Autodesk Inventor part; units mm, degrees
ref_plane "YZ Plane" through (0, 0, 0) normal (1, 0, 0) x (0, 1, 0)
ref_plane "XZ Plane" through (0, 0, 0) normal (0, 1, 0) x (-1, 0, 0)
ref_plane "XY Plane" through (0, 0, 0) normal (0, 0, 1) x (1, 0, 0)
sketch "Sketch1" plane through (0, 0, 0) normal (0, 0, 1) x (1, 0, 0)
  line L0 (13.75, -9.25) -> (-13.75, -9.25)
  line L1 (-13.75, -9.25) -> (-13.75, 9.25)
  line L2 (-13.75, 9.25) -> (13.75, 9.25)
  line L3 (13.75, 9.25) -> (13.75, -9.25)
  line L4 (13.75, -9.25) -> (-13.75, 9.25) construction
  line L5 (-13.75, -9.25) -> (13.75, 9.25) construction
  line L6 (-16, 0) -> (16, 0) construction
  circle A0 centre (-16, 0) radius 4
  circle A1 centre (16, 0) radius 4
  line L7 (30, -1) -> (-30, -1)
  line L8 (-30, -1) -> (-30, 1)
  line L9 (-30, 1) -> (30, 1)
  line L10 (30, 1) -> (30, -1)
  line L11 (30, -1) -> (-30, 1) construction
  line L12 (-30, -1) -> (30, 1) construction
  line L13 (30, -6.5) -> (-30, -6.5)
  line L14 (-30, -6.5) -> (-30, 6.5)
  line L15 (-30, 6.5) -> (30, 6.5)
  line L16 (30, 6.5) -> (30, -6.5)
  line L17 (30, -6.5) -> (-30, 6.5) construction
  line L18 (-30, -6.5) -> (30, 6.5) construction
  point P0 (0, 0)
  point P1 (-19.873, -1)
  point P2 (-13.75, -6.5)
  point P3 (13.75, -6.5)
  point P4 (19.873, -1)
  point P5 (19.873, 1)
  point P6 (13.75, 6.5)
  point P7 (-13.75, 6.5)
  point P8 (-19.873, 1)
  dimension "d0" = 27.5
  dimension "d1" = 18.5
  dimension "d2" = 8
  dimension "d3" = 8
  dimension "d4" = 32
  dimension "d5" = 60
  dimension "d6" = 2
  dimension "d7" = 13
extrude "Extrusion1" add sketch "Sketch1" along normal blind 6.35 contours L0 L1 L13 L3 | L13 L1 A0 L7 A1 L3 | L3 A1 L7 L16 L13 | L13 L14 L7 A0 L1 | L7 A0 L9 A1 | L9 A0 L1 L15 L3 A1 | L9 A1 L3 L15 L16 | L9 L14 L15 L1 A0 | L15 L1 L2 L3
fillet "Fillet4" radius 3 4 edges at (-19.873, 1, 3.175) (-19.873, -1, 3.175) (19.873, 1, 3.175) (19.873, -1, 3.175)
fillet "Fillet1" radius 2 4 edges at (13.75, 9.25, 3.175) (-13.75, 9.25, 3.175) (-13.75, -9.25, 3.175) (13.75, -9.25, 3.175)
fillet "Fillet2" radius 2 4 edges at (-30, 6.5, 3.175) (-30, -6.5, 3.175) (30, 6.5, 3.175) (30, -6.5, 3.175)
fillet "Fillet3" radius 1 8 edges at (-30, -1, 3.175) (-30, 1, 3.175) (-13.75, -6.5, 3.175) (-13.75, 6.5, 3.175) (13.75, 6.5, 3.175) (13.75, -6.5, 3.175) (30, 1, 3.175) (30, -1, 3.175)
sketch "Sketch2" plane through (0, 0, 6.35) normal (0, 0, 1) x (1, 0, 0)
  line L0 (10, -5.5) -> (-10, -5.5) construction
  line L1 (-10, -5.5) -> (-10, 5.5) construction
  line L2 (-10, 5.5) -> (10, 5.5) construction
  line L3 (10, 5.5) -> (10, -5.5) construction
  line L4 (10, -5.5) -> (-10, 5.5) construction
  line L5 (-10, -5.5) -> (10, 5.5) construction
  circle A0 centre (-10, 5.5) radius 3 construction
  circle A1 centre (-10, -5.5) radius 3 construction
  circle A2 centre (-10, 5.5) radius 1.65 construction
  line L6 (11.75, 9.25) -> (-11.75, 9.25) construction
  point P0 (0, 0)
  dimension "d13" = 20
  dimension "d14" = 11
  dimension "d22" = 6
  dimension "d23" = 6
  dimension "d25" = 3.3
  dimension "d26" = 2.1
hole "Hole1" at (-10, 5.5, 6.35) at (10, 5.5, 6.35) at (10, -5.5, 6.35) at (-10, -5.5, 6.35) direction (0, 0, -1) diameter 3.3 end through all
sketch "Sketch3" plane through (0, 0, 6.35) normal (0, 0, 1) x (1, 0, 0)
  point P0 (0, 0)
hole "Hole2" at (0, 0, 6.35) direction (0, 0, -1) diameter 3.3 end through all
properties part number "Printhead Belt Retainer R2" material "Aluminum 6061"
Can you work these out from the model? Positions are in its coordinate system, mm. A direction names the side the tool comes from. Coordinates: 2 decimals unless noted, no trailing zeros. Write each loop counter-clockwise with the first axis right and the second up, starting at its lowest first coordinate (ties: lowest second). Pieces come first, ordered by that corner, then holes. Notation, with made-up numbers: (77.5, -9) - (131.5, -9) arc R27 ccw to (131.5, 22) - close; hole circle Ø1 at (75.25, 49). An arc over 180 degrees is marked (long way). Return JSON: item names as keys, results as strings.
Q1. If we section it at A-A (y = 0): Please give me the cut outline in (x, z).
Computed values:
{"outline": "(-12, 0) - (-1.65, 0) - (-1.65, 6.35) - (-12, 6.35) - close; (1.65, 0) - (12, 0) - (12, 6.35) - (1.65, 6.35) - close"}
Q2. Please list where these lines run through material, in increasing order: L1, parallel to Y at x = 22.5, z = 3.25; L2, parallel to Y at x = 10, z = 3.5; L3, parallel to X at y = -5.5, z = 2.75. Write a range as from..to.
Computed values:
{"L1": "y = -6.5..-1, 1..6.5", "L2": "y = -9.25..-7.15, -3.85..3.85, 7.15..9.25", "L3": "x = -29.73..-11.65, -8.35..8.35, 11.65..29.73"}
Q3. I'm going to push flat-ended pins straight in: pin 1 Ø5 at (x, y) = (-16, 0) entering from -Z; pin 2 Ø1.9 at (x, z) = (21, 3) entering from +Y; pin 3 Ø1.5 at (y, z) = (0, 4.5) entering from +X. Where does each tip first touch, or does it pass through?
Computed values:
{"pin 1": "passes through", "pin 2": "stops at y = 6.5", "pin 3": "stops at x = 12.07"}
Q4. If we section it at B-B (x = -16): Please give me the cut outline in (y, z).
Computed values:
{"outline": "(-6.5, 0) - (-4, 0) - (-4, 6.35) - (-6.5, 6.35) - close; (4, 0) - (6.5, 0) - (6.5, 6.35) - (4, 6.35) - close"}
Q5. If we section it at D-D (y = -5.5): Please give me the cut outline in (x, z).
Computed values:
{"outline": "(-29.73, 0) - (-11.65, 0) - (-11.65, 6.35) - (-29.73, 6.35) - close; (-8.35, 0) - (8.35, 0) - (8.35, 6.35) - (-8.35, 6.35) - close; (11.65, 0) - (29.73, 0) - (29.73, 6.35) - (11.65, 6.35) - close"}
Q6. Thinking about a two-plate mould opening in Y: for faces 1 (the flat face through (-30, -3, 3)), 2 (the cylindrical face through (29.715, -1.301, 3.219)), 3 (the cylindrical face through (29.699, 1.285, 3.219)), 4 (the cylindrical face through (-29.43, -5.9, 3.22)), which applies, +Y half, -Y half, draft (parallel to the pull), parting line (faces both ways), or undercut?
Computed values:
{"face 1": "draft", "face 2": "undercut", "face 3": "undercut", "face 4": "-Y half"}
Q7. If we section it at C-C (x = 10): Please give me the cut outline in (y, z), then the cut area to 3 significant figures.
Computed values:
{"outline": "(-9.25, 0) - (-7.15, 0) - (-7.15, 6.35) - (-9.25, 6.35) - close; (-3.85, 0) - (3.85, 0) - (3.85, 6.35) - (-3.85, 6.35) - close; (7.15, 0) - (9.25, 0) - (9.25, 6.35) - (7.15, 6.35) - close", "area": "75.6 mm2"}
Q8. On a 3-axis mill with a long thin cutter (end or side, diameter ignored), from which of +Z, -Z, +X, -X, +Y, -Y can I reach the whole of each face in a straight line? I mean faces 5 (the flat face through (21, 6.5, 3)), 6 (the cylindrical face through (-29.699, -1.285, 3.219)), 7 (the flat face through (25, -1, 3)). Say none if no direction works.
Computed values:
{"face 5": "+Z, -Z, +X, +Y", "face 6": "+Z, -Z, -X", "face 7": "+Z, -Z, +X"}
